Autodesk Inventor part; units mm, degrees
ref_plane "YZ Plane" through (0, 0, 0) normal (1, 0, 0) x (0, 1, 0)
ref_plane "XZ Plane" through (0, 0, 0) normal (0, 1, 0) x (-1, 0, 0)
ref_plane "XY Plane" through (0, 0, 0) normal (0, 0, 1) x (1, 0, 0)
sketch "Esboço1" plane through (0, 0, 0) normal (0, 1, 0) x (-1, 0, 0)
  arc A0 (-221.4815, -24.8392) -> (-98.2625, -26.3329) centre (-159.863, -24.8392) ccw
  arc A1 (-72.9226, -1.6) -> (-98.2625, -26.3329) centre (-72.9226, -26.9474) ccw
  line L0 (-72.9226, -1.6) -> (-35, -1.6)
  arc A2 (-35, -68.4) -> (-35, -1.6) centre (-35, -35) ccw
  arc A3 (-35, -68.4) -> (-47.9358, -81.3358) centre (-35, -81.3358) ccw
  arc A4 (-35, -50.4) -> (-65.9358, -81.3358) centre (-35, -81.3358) ccw
  arc A5 (-35, -50.4) -> (-35, -19.6) centre (-35, -35) ccw
  line L1 (-35, -19.6) -> (-72.9226, -19.6)
  arc A6 (-72.9226, -19.6) -> (-80.2678, -26.7693) centre (-72.9226, -26.9474) ccw
  arc A7 (-239.4815, -24.8392) -> (-80.2678, -26.7693) centre (-159.863, -24.8392) ccw
  arc A8 (-241.0815, -24.8392) -> (-78.6683, -26.808) centre (-159.863, -24.8392) ccw
  arc A9 (-72.9226, -21.2) -> (-78.6683, -26.808) centre (-72.9226, -26.9474) ccw
  line L2 (-72.9226, -21.2) -> (-35, -21.2)
  arc A10 (-35, -48.8) -> (-35, -21.2) centre (-35, -35) ccw
  arc A11 (-35, -48.8) -> (-67.5358, -81.3358) centre (-35, -81.3358) ccw
  arc A12 (-219.8815, -24.8392) -> (-99.8621, -26.2941) centre (-159.863, -24.8392) ccw
  arc A13 (-72.9226, 0) -> (-99.8621, -26.2941) centre (-72.9226, -26.9474) ccw
  line L3 (-72.9226, 0) -> (-35, 0)
  arc A14 (-35, -70) -> (-35, 0) centre (-35, -35) ccw
  arc A15 (-35, -70) -> (-46.3358, -81.3358) centre (-35, -81.3358) ccw
  line L4 (-219.8815, -24.8392) -> (-241.0815, -24.8392)
  line L5 (-46.3358, -81.3358) -> (-67.5358, -81.3358)
  line L6 (-78.6718, -26.9474) -> (-80.2724, -26.9474)
  line L7 (-99.8815, -26.9474) -> (-98.2805, -26.9474)
  line L8 (-35, -1.6) -> (-35, 0)
  line L9 (-35, -70) -> (-35, -68.4)
  line L10 (-72.9226, -1.6) -> (-72.9226, 0)
  point P0 (0, 0)
  point P1 (-53.9613, -19.6)
  point P2 (-35, -69.2)
  point P3 (-35, -0.8)
  point P4 (-79.4721, -26.9474)
  point P5 (-99.081, -26.9474)
  point P6 (-239.4815, -24.8392)
  point P7 (-35, -68.4)
  point P8 (-35, -70)
  point P9 (0, -35)
  point P10 (-53.9613, 0)
  dimension "d10" = 18
  dimension "d11" = 30.8
  dimension "d12" = 1.6
  dimension "d13" = 1.6
  dimension "d21" = 120
extrude "Extrusão1" add sketch "Esboço1" against normal blind 1.6
extrude "Extrusão2" add sketch "Esboço1" along normal blind 18 contours L7 A12 A13 L10 A1 A0 | A7 L6 A8 L4 | L8 A14 L9 A2
extrude "Extrusão3" add sketch "Esboço1" along normal blind 9 contours L4 A12 L7 A0 | A7 A6 L1 A5 A4 L5 A11 A10 L2 A9 A8 L6 | L10 L3 L8 L0 | L9 A15 L5 A3
fillet "Arredondamento1" radius 9 8 edges at (78.0546, 0, -21.6894) (53.9613, 0, -19.6) (19.6, 0, -35) (56.8749, 0, -59.4609) (160.828, 0, -104.4519) (90.6273, 0, -8.8081) (1.6, 0, -35) (53.9613, 0, -1.6)
equation "\"d10\" = Esfera"
equation "\"d12\" = Margem"
equation "\"d13\" = Margem"
equation "\"Esfera\" = 18"
equation "\"Margem\" = 1.6"
properties part number "Agrupar bolinhas novamente"
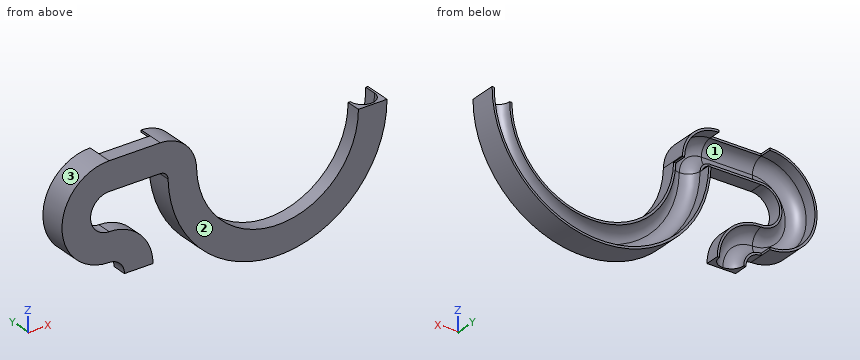
The listing builds one solid part. Answer for the finished solid, in the listing's coordinates (mm). Face numbers are marked on the shaded views. Coordinates: 2 decimals unless noted, no trailing zeros. Loops run counter-clockwise (first coordinate to the right, second up) from the corner with the lowest first, then second, coordinate; pieces in that order, holes last. Notation, with made-up numbers: M 32,74.25 L 64,74.25 A11 cw 64,93.25 Z; hole C 39.25,-6.75 d4. An arc over 180 degrees is marked long. Answer in a Markdown table with one row per item.
1) Determine the mould class of the marked faces 1, 2 and 3 for opening direction X: released by +X, released by -X, zero draft, split by the parting line, or undercut.
Answers below:
| item | result |
|---|---|
| face 1 | undercut |
| face 2 | zero draft |
| face 3 | released by -X |
2) Find section A-A (y = 15.5). Determine the outline of the cut face in (x, z), then the cut area to 3 significant figures.
Answers below:
| item | result |
|---|---|
| outline | M 35,-70 L 35,-68.4 A33.4 cw 35,-1.6 L 35,0 A35 ccw Z; M 72.92,-1.6 A25.35 cw 98.26,-26.33 A61.62 ccw 98.28,-26.95 L 99.88,-26.95 A60.02 cw 99.86,-26.29 A26.95 ccw 72.92,0 Z; M 78.67,-26.95 A81.22 ccw 241.08,-24.84 L 239.48,-24.84 A79.62 cw 80.27,-26.95 Z |
| area | 638 mm^2 |
3) Given pin 1 (2 mm diameter, centred on x = 140, y = 9.5, fed in from +Z); pin 2 (3 mm diameter, centred on x = 192.5, y = 13.5, fed in from +Z); pin 3 (8 mm diameter, centred on y = 1, z = -56.5, fed in from -X), each flat-ended and moving along its own axis, determine where each tip first touches the part or whether it passes through.
Answers below:
| item | result |
|---|---|
| pin 1 | z = -81.16 |
| pin 2 | z = -96.77 |
| pin 3 | x = 4.69 |
4) Find the intervals of material crossed by probe 1 along X at (y, z) = (13.25, -35); probe 2 along X at (y, z) = (11.25, -38.5); probe 3 along X at (y, z) = (5, -25), in increasing order.
Answers below:
| item | result |
|---|---|
| probe 1 | 0 to 1.6, 79.28 to 80.9, 238.83 to 240.44 |
| probe 2 | 0.18 to 1.78, 79.8 to 81.43, 238.3 to 239.92 |
| probe 3 | 1.46 to 4.12, 22.08 to 25.49, 78.33 to 80.98, 97.25 to 99.8, 219.88 to 222.42, 238.54 to 241.08 |
